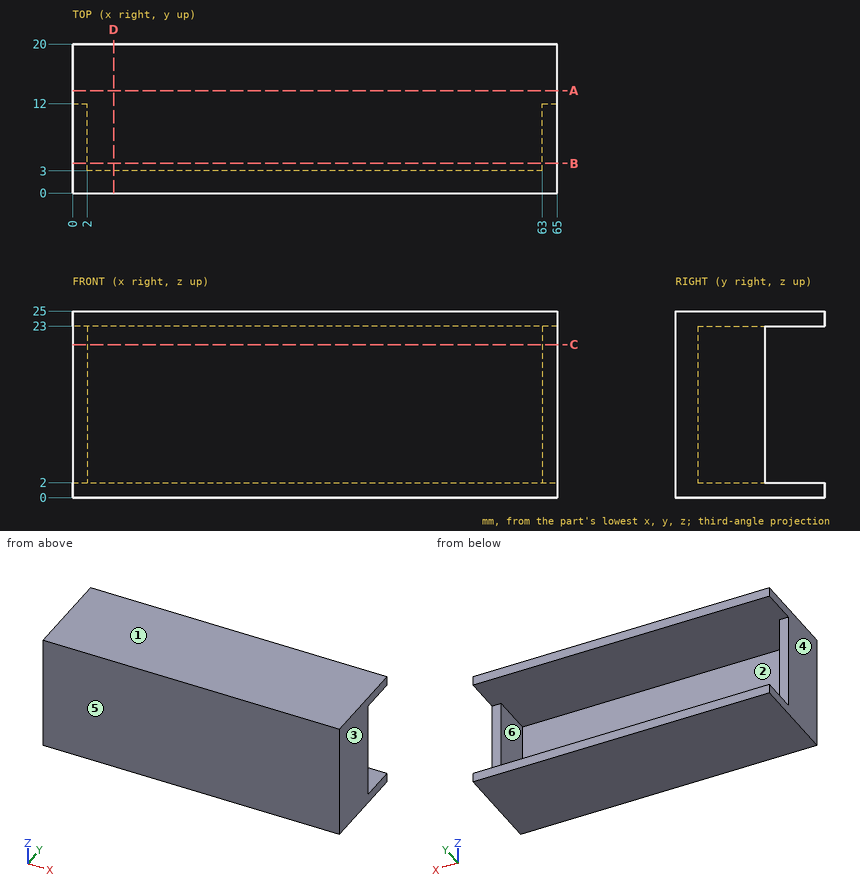
The drawing under review shows one solid part. Ordinate dimensions are in mm from its lowest x, y, z. A direction names the side the tool comes from. Give positions to 0.01 mm unless a question says otherwise; leave off trailing zeros. Order: outer loops, then holes, each group sorted by start corner. A loop starts at its lowest first (then second) coordinate and runs counter-clockwise, first axis right, second up. Notation, with made-up numbers: M 56,-10.5 L 105,-10.5 A20 ccw 105,0.5 Z; hole C -3,19.5 d5. An arc over 180 degrees is marked long. Answer in a Markdown table with one row per item. Add a question column.
1. For pin 1 Ø10.5 at (x, z) = (37.5, 10.5) entering from +Y; pin 2 Ø1.5 at (y, z) = (17, 21.5) entering from +X; pin 3 Ø1.6 at (x, z) = (64, 8.5) entering from +Y, all flat-tipped, find the tip position at first contact; note any pin that passes through.
2. To check wall thickness, follow line 1 along Z through (x, y) = (37.5, 5.25); line 2 along X through (y, z) = (4.25, 12.5); line 3 along Y through (x, z) = (33, 7.5). State the ranges of each line that lie inside material, in increasing order.
3. Machinability: for the marked faces 5 and 6, which of the approach directions +Z, -Z, +X, -X, +Y, -Y give a long, thin tool a straight path to every point of the face, cutting with its end or side? Answer none if there is none.
4. Add section C-C on z = 20.5. State the section outline as (x, y) points.
5. Mouldability with a two-part tool opening along X and no side actions: class the marked faces 1, 2, 3 and 4 as released by +X, released by -X, zero draft, split by the parting line, or undercut.
6. Add section A-A on y = 13.75. State the section outline as (x, z) points, plus the area to 3 significant figures.
7. Add section D-D on x = 5.5. State the section outline as (y, z) points, plus the area to 3 significant figures.
8. Add section B-B on y = 4. State the section outline as (x, z) points, plus the area to 3 significant figures.
The answers:
| question | item | result |
|---|---|---|
| 1 | pin 1 | y = 3 |
| 1 | pin 2 | through |
| 1 | pin 3 | y = 12 |
| 2 | line 1 | 0 to 2, 23 to 25 |
| 2 | line 2 | 0 to 2, 63 to 65 |
| 2 | line 3 | 0 to 3 |
| 3 | face 5 | +Z, -Z, +X, -X, -Y |
| 3 | face 6 | +Y |
| 4 | outline | M 0,0 L 65,0 L 65,12 L 63,12 L 63,3 L 2,3 L 2,12 L 0,12 Z |
| 5 | face 1 | zero draft |
| 5 | face 2 | undercut |
| 5 | face 3 | released by +X |
| 5 | face 4 | released by -X |
| 6 | outline | M 0,0 L 65,0 L 65,2 L 0,2 Z; M 0,23 L 65,23 L 65,25 L 0,25 Z |
| 6 | area | 260 mm2 |
| 7 | outline | M 0,0 L 20,0 L 20,2 L 3,2 L 3,23 L 20,23 L 20,25 L 0,25 Z |
| 7 | area | 143 mm2 |
| 8 | outline | M 0,0 L 65,0 L 65,25 L 0,25 Z; hole M 2,2 L 63,2 L 63,23 L 2,23 Z |
| 8 | area | 344 mm2 |
